Geometry check sheet. Reference: the model listing, model coordinates, mm. Face numbers are marked on the shaded views. Round coordinates to 2 decimals unless told otherwise and drop trailing zeros. Order: outer loops, then holes, each group sorted by start corner. A loop starts at its lowest first (then second) coordinate and runs counter-clockwise, first axis right, second up.
```python
from build123d import *

# Parameters (mm, degrees)
ESQUISSE1_R             = 1.6
ESQUISSE1_W             = 5
ESQUISSE1_H             = 20
ESQUISSE1_W_2           = 20
ESQUISSE1_H_2           = 5
BOSS_EXTRU_1_DEPTH      = 5
CONG_1_R                = 10
ESQUISSE2_R             = 4
ESQUISSE2_R_2           = 1.625
ENL_V_MAT_EXTRU_1_DEPTH = 10


with BuildPart() as part:
    # Esquisse1 → Boss.-Extru.1 (new body)
    with BuildSketch(Plane.XY):
        Polygon((-55, 35), (55, 35), (55, -35), (25, -35), (25, -40), (10, -40), (10, -35), (5, -35), (5, -30), (-5, -30), (-5, -35), (-10, -35), (-10, -40), (-25, -40), (-25, -35), (-55, -35), align=None)
        with Locations((-25, 17.5)):
            Circle(ESQUISSE1_R, mode=Mode.SUBTRACT)
        with Locations((25, 17.5)):
            Circle(ESQUISSE1_R, mode=Mode.SUBTRACT)
        with Locations((-30, -10)):
            Rectangle(ESQUISSE1_W, ESQUISSE1_H, mode=Mode.SUBTRACT)
        with Locations((30, -10)):
            Rectangle(ESQUISSE1_W, ESQUISSE1_H, mode=Mode.SUBTRACT)
        with Locations((0, 17.5)):
            Rectangle(ESQUISSE1_W_2, ESQUISSE1_H_2, mode=Mode.SUBTRACT)
    extrude(amount=BOSS_EXTRU_1_DEPTH)

    # Congé1
    cong_1_edges = [part.edges().sort_by_distance(p)[0] for p in [
        (-55, 35, 2.5),
        (55, 35, 2.5),
    ]]
    fillet(cong_1_edges, radius=CONG_1_R)

    # Esquisse2 → Enlèv. mat.-Extru.1 (cut)
    with BuildSketch(Plane(origin=(0, 0, 0), x_dir=(-1, 0, 0), z_dir=(0, 0, -1))):
        with Locations((-45, 25)):
            Circle(ESQUISSE2_R)
        with Locations((-50.303300859, 19.696699141)):
            Circle(ESQUISSE2_R_2)
        with Locations((-39.696699141, 30.303300859)):
            Circle(ESQUISSE2_R_2)
    enl_v_mat_extru_1 = extrude(amount=-ENL_V_MAT_EXTRU_1_DEPTH, mode=Mode.SUBTRACT)

    # Symétrie1: Enlèv. mat.-Extru.1 across plane
    add(enl_v_mat_extru_1.mirror(Plane(origin=(0, 0, 0), x_dir=(0, 0, 1), z_dir=(1, 0, 0))), mode=Mode.SUBTRACT)


solid = part.part
```
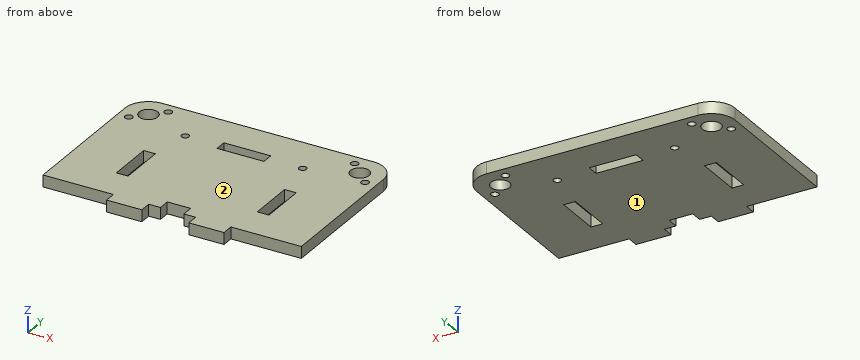
(1) Material ranges on line 1 (X direction, y = -19, z = 2); line 2 (Y direction, x = -8, z = 0.7); line 3 (Y direction, x = -1.5, z = 2.3), recorded low to high.
Returned:
line 1: x = -55 to -32.5, -27.5 to 27.5, 32.5 to 55
line 2: y = -35 to 15, 20 to 35
line 3: y = -30 to 15, 20 to 35
(2) Draft check along Z on the marked faces 1 and 2. Enter one of: released by +Z, released by -Z, zero draft, split by the parting line, or undercut.
Returned:
face 1: released by -Z
face 2: released by +Z
(3) Depth check by flat-ended pin: P1, Ø5, axis at x = 32, y = -12, coming from the -Z side; P2, Ø5, axis at x = 45, y = 25, coming from the +Z side; P3, Ø2.5, axis at x = 8, z = 3, coming from the -Y side; P4, Ø1.5, axis at x = -0.5, z = 1.5, coming from the -Y side. Enter the tip coordinate at first touch or a pass-through.
Returned:
P1: stops at z = 0
P2: passes through
P3: stops at y = -35
P4: stops at y = -30
(4) Sectioned sample at A-A, the plane x = -37. Record the cut outline in (y, z).
Returned:
outline: (-35, 0) - (35, 0) - (35, 5) - (-35, 5) - close
(5) Sectioned sample at B-B, the plane z = 1.5. Give the number of separate pieces and of enclosed holes in the cut face, and give its area (3 significant figures).
Returned:
separate pieces: 1
enclosed holes: 11
area: 7,310 mm2
